For this review, use the dimensioned drawing (mm, ordinates from the lowest corner) and the shaded views. A direction names the side the tool comes from. Round coordinates to 2 decimals unless told otherwise and drop trailing zeros. Loops run counter-clockwise (first coordinate to the right, second up) from the corner with the lowest first, then second, coordinate; pieces in that order, holes last. Notation, with made-up numbers: M 30,23 L 81,23 A25 cw 81,58 Z; hole C 44,13.25 d11. An arc over 180 degrees is marked long. Answer as a JSON object with one key per item and string values. Group by question number.
Item 1: The part is to be moulded in two halves that separate along Y. For the marked faces 1, 2, 3 and 4, say which applies: +Y half, -Y half, draft (parallel to the pull), parting line (faces both ways), or undercut.
Item 2: Consider section C-C (x = 33.5). Give the boundary of the cut face in (y, z).
Item 3: Consider section A-A (z = 10.5). State how many separate pieces and enclosed holes the cut face has, and give its area (3 significant figures).
Item 4: Consider section B-B (y = 6). Give the boundary of the cut face in (x, z) (3 decimals).
Item 5: Consider section D-D (y = 2.75). Give the boundary of the cut face in (x, z), and give its area (3 significant figures).
Item 6: To check wall thickness, follow line 1 (Y direction, x = 4, z = 9); line 2 (X direction, y = 6.25, z = 10.75); line 3 (X direction, y = 3.5, z = 4.5). State the ranges of each line that lie inside material, in increasing order.
Item 7: Insertion check: P1, Ø2, axis at x = 17, y = 2, coming from the -Z side; P2, Ø4, axis at y = 1.5, z = 7, coming from the +X side; P3, Ø0.5, axis at y = 0.5, z = 10, coming from the +X side; P4, Ø1.5, axis at y = 1.5, z = 9.5, coming from the -X side. Each pin has a flat end and moves straight along its axis. Give the tip position at first contact, or say it passes through.
Item 8: Tool access review of the marked faces 5, 6 and 7: name each direction out of +Z, -Z, +X, -X, +Y, -Y from which nothing blocks a thin tool from reaching the whole face with its end or side.
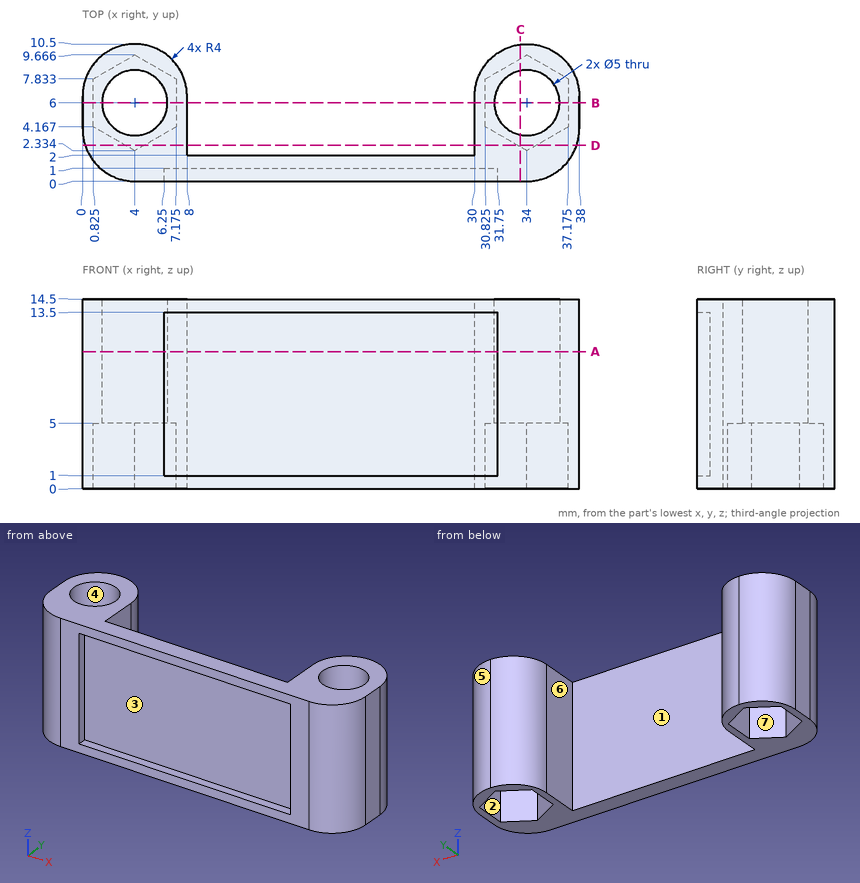
Geometry results:
{
 "1": {"face 1": "+Y half", "face 2": "undercut", "face 3": "-Y half", "face 4": "undercut"},
 "2": {"outline": "M 0,0 L 2.62,0 L 2.62,5 L 3.55,5 L 3.55,14.5 L 0,14.5 Z; M 8.45,5 L 9.38,5 L 9.38,0 L 10.47,0 L 10.47,14.5 L 8.45,14.5 Z"},
 "3": {"separate pieces": "1", "enclosed holes": "2", "area": "127 mm^2"},
 "4": {"outline": "M 0,0 L 0.825,0 L 0.825,5 L 1.5,5 L 1.5,14.5 L 0,14.5 Z; M 6.5,5 L 7.175,5 L 7.175,0 L 8,0 L 8,14.5 L 6.5,14.5 Z; M 30,0 L 30.825,0 L 30.825,5 L 31.5,5 L 31.5,14.5 L 30,14.5 Z; M 36.5,5 L 37.175,5 L 37.175,0 L 38,0 L 38,14.5 L 36.5,14.5 Z"},
 "5": {"outline": "M 0.2,0 L 3.28,0 L 3.28,5 L 4.72,5 L 4.72,0 L 8,0 L 8,14.5 L 0.2,14.5 Z; M 30,0 L 33.28,0 L 33.28,5 L 34.72,5 L 34.72,0 L 37.8,0 L 37.8,14.5 L 30,14.5 Z", "area": "212 mm^2"},
 "6": {"line 1": "y = 0 to 3.5, 8.5 to 10.5", "line 2": "x = 0 to 1.51, 6.49 to 8, 30 to 31.51, 36.49 to 38", "line 3": "x = 0.03 to 1.98, 6.02 to 8, 30 to 31.98, 36.02 to 37.97"},
 "7": {"P1": "stops at z = 0", "P2": "stops at x = 37.97", "P3": "stops at x = 36.33", "P4": "stops at x = 0.4"},
 "8": {"face 5": "+Z, -Z, +X, +Y", "face 6": "+Z, -Z, +Y", "face 7": "-Z"}
}
